Part model, mm, in its own coordinate system. Face numbers are marked on the shaded views. A direction names the side the tool comes from. Round coordinates to 2 decimals unless told otherwise and drop trailing zeros. Order: outer loops, then holes, each group sorted by start corner. A loop starts at its lowest first (then second) coordinate and runs counter-clockwise, first axis right, second up. Notation, with made-up numbers: M 80,63 L 97,63 A19 cw 97,79 Z; hole C 7,50 d7. An arc over 180 degrees is marked long. One line per question, with ' | ' between items.
from build123d import *

# Parameters (mm, degrees)
F0_R     = 3
F0_R_2   = 4.5
F1_DEPTH = 8
F2_R     = 10
F4_DEPTH = 4.5
F5_SIZE2 = 4.49999
F5_SIZE  = 1.99999


# Not quite as in the source:
# - a fillet or chamfer is up to 0.001 mm smaller than in the source, because OpenCascade refuses the exact size


with BuildPart() as f1:
    # F0 (on Front) → F1 (new body)
    with BuildSketch(Plane.XZ):
        with BuildLine():
            ThreePointArc((-6.9538789093, 27.1904505494), (1.4310674653, 22.6377961241), (7.5, 30))
            ThreePointArc((7.5, 30), (6.2613081918, 34.1286825656), (2.9543947393, 36.8935877251))
            ThreePointArc((2.9543947393, 36.8935877251), (-5.247540964, 35.3584805524), (-6.9538789093, 27.1904505494))
        make_face()
        with Locations((0, 30)):
            Circle(F0_R, mode=Mode.SUBTRACT)
        with BuildLine():
            ThreePointArc((2.9543947393, 36.8935877251), (6.2613081918, 34.1286825656), (7.5, 30))
            ThreePointArc((7.5, 30), (1.4310674653, 22.6377961241), (-6.9538789093, 27.1904505494))
            Line((-6.9538789093, 27.1904505494), (4.031776205, 0))
            Line((4.031776205, 0), (-6.9538789093, -27.1904505494))
            ThreePointArc((-6.9538789093, -27.1904505494), (1.4310674653, -22.6377961241), (7.5, -30))
            ThreePointArc((7.5, -30), (6.2613081918, -34.1286825656), (2.9543947393, -36.8935877251))
            Line((2.9543947393, -36.8935877251), (72.9543947393, -6.8935877251))
            ThreePointArc((72.9543947393, -6.8935877251), (62.5, 0), (72.9543947393, 6.8935877251))
            Line((72.9543947393, 6.8935877251), (2.9543947393, 36.8935877251))
        make_face()
        with BuildLine():
            ThreePointArc((77.5, 0), (76.2613081918, 4.1286825656), (72.9543947393, 6.8935877251))
            ThreePointArc((72.9543947393, 6.8935877251), (62.5, 0), (72.9543947393, -6.8935877251))
            ThreePointArc((72.9543947393, -6.8935877251), (76.2613081918, -4.1286825656), (77.5, 0))
        make_face()
        with Locations((70, 0)):
            Circle(F0_R_2, mode=Mode.SUBTRACT)
        with BuildLine():
            ThreePointArc((7.5, -30), (1.4310674653, -22.6377961241), (-6.9538789093, -27.1904505494))
            ThreePointArc((-6.9538789093, -27.1904505494), (-5.247540964, -35.3584805524), (2.9543947393, -36.8935877251))
            ThreePointArc((2.9543947393, -36.8935877251), (6.2613081918, -34.1286825656), (7.5, -30))
        make_face()
        with Locations((0, -30)):
            Circle(F0_R, mode=Mode.SUBTRACT)
    extrude(amount=F1_DEPTH)

    # F2
    f2_edges = [f1.edges().sort_by_distance(p)[0] for p in [
        (4.031776, -4, 0),
    ]]
    fillet(f2_edges, radius=F2_R)

    # F3 (on Front) → F4 (cut)
    with BuildSketch(Plane.XZ):
        with BuildLine():
            Line((12.5995942419, 16.7481284808), (17.8527685007, 3.7460659342))
            ThreePointArc((17.8527685007, 3.7460659342), (18.580929955, 0), (17.8527685007, -3.7460659342))
            Line((17.8527685007, -3.7460659342), (12.5995942419, -16.7481284808))
            ThreePointArc((12.5995942419, -16.7481284808), (13.0546176939, -18.926269815), (15.2418005482, -19.3356317277))
            Line((15.2418005482, -19.3356317277), (53.9242593693, -2.7574350901))
            ThreePointArc((53.9242593693, -2.7574350901), (55.7425014736, 0), (53.9242593693, 2.7574350901))
            Line((53.9242593693, 2.7574350901), (15.2418005482, 19.3356317277))
            ThreePointArc((15.2418005482, 19.3356317277), (13.0546176939, 18.926269815), (12.5995942419, 16.7481284808))
        make_face()
    extrude(amount=F4_DEPTH, mode=Mode.SUBTRACT)

    # F5 (size 2 and 4.5 in the source; OpenCascade refuses exactly that, so slightly less here)
    f5_edges = [f1.edges().sort_by_distance(p)[0] for p in [
        (34.58303, -4.5, 11.046533),
    ]]
    f5_side = f1.faces().sort_by_distance((30.018515, -4.5, 0))[0]
    chamfer(f5_edges, length=F5_SIZE, length2=F5_SIZE2, reference=f5_side)


solid = f1.part
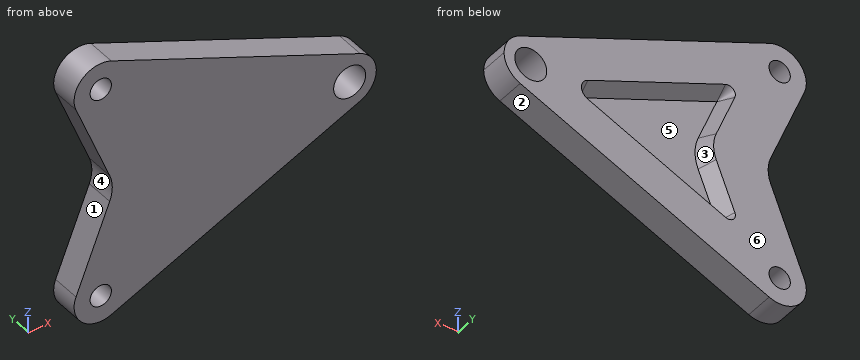
1) Drop flat-ended pins along their axis: pin 1 (10.5 mm diameter, centred on x = 27.5, z = -4, fed in from +Y); pin 2 (2 mm diameter, centred on y = -6, z = 27.5, fed in from +X); pin 3 (7 mm diameter, centred on x = 70, z = 0, fed in from -Y); pin 4 (2 mm diameter, centred on x = 35.5, y = -7, fed in from -Z). Give the stop position or say it passes through.
The answers:
pin 1: stops at y = -4.5 | pin 2: stops at x = 27.21 | pin 3: passes through | pin 4: stops at z = -23.37
2) Two-plate mould, pull along X, no slides. Class the marked faces 4, 5 and 6: released by +X, released by -X, zero draft, split by the parting line, or undercut.
The answers:
face 4: released by -X | face 5: undercut | face 6: zero draft
3) Saw through at B-B (x = 0). List the corners of the cut face in (y, z), plus the area to 3 significant figures.
The answers:
outline: M -8,-37.5 L 0,-37.5 L 0,-33 L -8,-33 Z; M -8,-27 L 0,-27 L 0,-9.98 L -8,-9.98 Z; M -8,9.98 L 0,9.98 L 0,27 L -8,27 Z; M -8,33 L 0,33 L 0,37.5 L -8,37.5 Z | area: 344 mm²
4) Probe line 1 (Z direction, x = 0, y = -2); line 2 (Z direction, x = 69, y = -5.5); line 3 (Z direction, x = 70, y = -1.5). List the from-to ranges inside material, lowest first. Write a range as [from, to].
The answers:
line 1: z = [-37.5, -33], [-27, -9.98], [9.98, 27], [33, 37.5] | line 2: z = [-8.59, -4.39], [4.39, 8.59] | line 3: z = [-8.16, -4.5], [4.5, 8.16]
5) Which spindle directions (+Z, -Z, +X, -X, +Y, -Y) get a long thin tool onto all of the face, cutting with end or side? Do the marked faces 1, 2 and 3. Say none if no direction does.
The answers:
face 1: -X, +Y, -Y | face 2: -Z, +X, +Y, -Y | face 3: +Y
6) Saw through at A-A (y = -6). List the corners of the cut face in (x, z).
The answers:
outline: M -6.95,-27.19 A7.5 ccw 2.95,-36.89 L 72.95,-6.89 A7.5 ccw 72.95,6.89 L 2.95,36.89 A7.5 ccw -6.95,27.19 L 2.52,3.75 A10 cw 2.52,-3.75 Z; hole C 0,-30 d6; hole C 0,30 d6; hole C 70,0 d9
7) Saw through at C-C (z = -29). List the corners of the cut face in (x, y), plus the area to 3 significant figures.
The answers:
outline: M -7.43,-8 L -2.83,-8 L -2.83,0 L -7.43,0 Z; M 2.83,-8 L 21.37,-8 L 21.37,0 L 2.83,0 Z | area: 185 mm²
